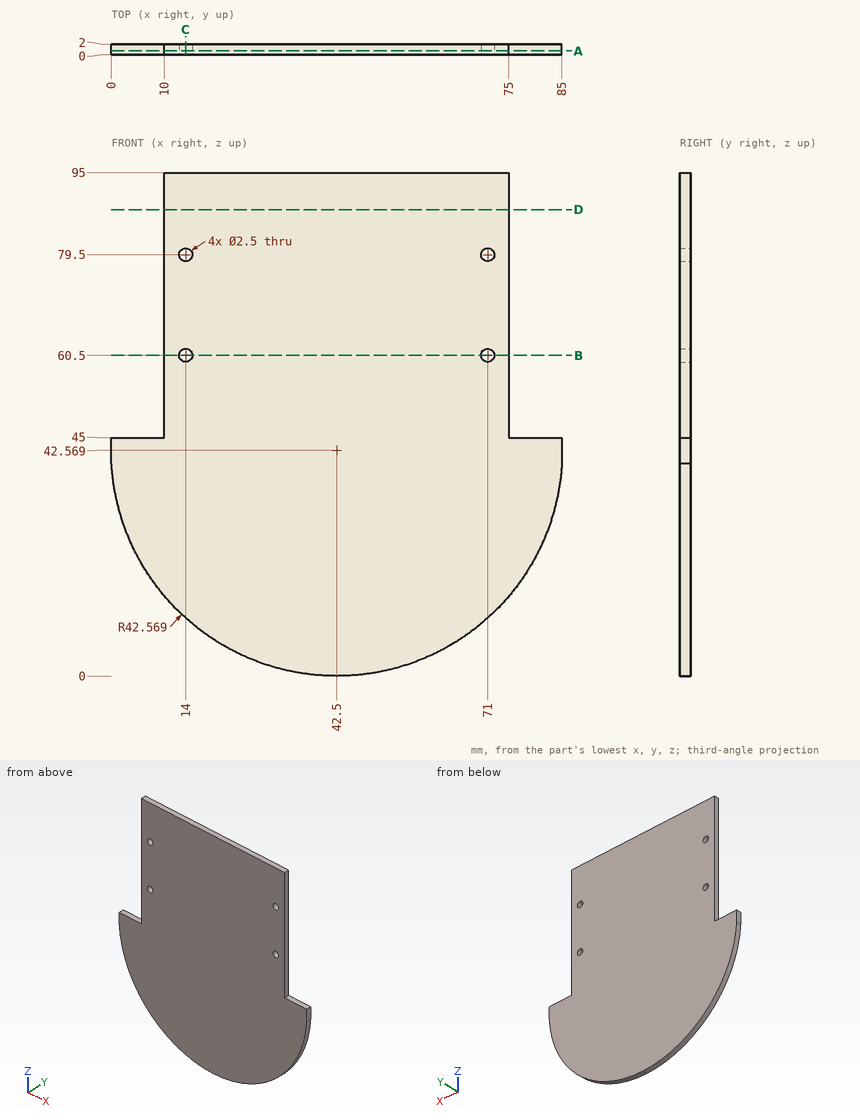
Check sheet for the drawn part. Datum: minimum x, y, z corner. Units: mm. Round coordinates to 2 decimals unless told otherwise and drop trailing zeros. Loops run counter-clockwise (first coordinate to the right, second up) from the corner with the lowest first, then second, coordinate; pieces in that order, holes last. Notation, with made-up numbers: M 86,31.25 L 133,31.25 A8 ccw 133,36.25 Z; hole C 87,-39 d8. An arc over 180 degrees is marked long. One line per question, with ' | ' between items. Start each with the question number.
Item 1: Scan lines: probe 1 along X at (y, z) = (1.3, 79.5); probe 2 along X at (y, z) = (0.6, 60) (1 decimal); probe 3 along Z at (x, y) = (14.5, 0.65) (1 decimal). Record each from-to range of solid material in increasing order.
Item 2: Gauge pin test, flat ends, axial feed: pin 1 Ø0.6 at (x, y) = (7.5, 1.5) entering from +Z; pin 2 Ø1 at (y, z) = (1.5, 62.5) entering from -X. Record the tip position at first contact, or that the pin passes through.
Item 3: Section check B-B (z = 60.5). Record the boundary of the cut face in (x, y), and give its area (3 significant figures).
Item 4: Section check C-C (x = 14). Record the boundary of the cut face in (y, z).
Item 5: Section check D-D (z = 88). Record the boundary of the cut face in (x, y).
Item 6: Section check A-A (y = 0.7). Record the boundary of the cut face in (x, z), and give its area (3 significant figures).
Worked out:
1) probe 1: 10 to 12.75, 15.25 to 69.75, 72.25 to 75 | probe 2: 10 to 12.9, 15.1 to 69.9, 72.1 to 75 | probe 3: 10.5 to 59.4, 61.6 to 78.4, 80.6 to 95
2) pin 1: z = 45 | pin 2: x = 10
3) outline: M 10,0 L 12.75,0 L 12.75,2 L 10,2 Z; M 15.25,0 L 69.75,0 L 69.75,2 L 15.25,2 Z; M 72.25,0 L 75,0 L 75,2 L 72.25,2 Z | area: 120 mm^2
4) outline: M 0,10.95 L 2,10.95 L 2,59.25 L 0,59.25 Z; M 0,61.75 L 2,61.75 L 2,78.25 L 0,78.25 Z; M 0,80.75 L 2,80.75 L 2,95 L 0,95 Z
5) outline: M 10,0 L 75,0 L 75,2 L 10,2 Z
6) outline: M 0,40.14 A42.57 ccw 85,40.14 L 85,45 L 75,45 L 75,95 L 10,95 L 10,45 L 0,45 Z; hole C 14,60.5 d2.5; hole C 14,79.5 d2.5; hole C 71,60.5 d2.5; hole C 71,79.5 d2.5 | area: 6,280 mm^2
